Model file for the job. Use its own axes, mm. A direction names the side the tool comes from. Coordinates: 2 decimals unless noted, no trailing zeros. Write each loop counter-clockwise with the first axis right and the second up, starting at its lowest first coordinate (ties: lowest second). Pieces come first, ordered by that corner, then holes. Notation, with made-up numbers: M 74,80.5 L 82,80.5 A23 cw 82,102.5 Z; hole C 87,12 d4. An arc over 180 degrees is marked long. Put each result on its own line as item: value. Start each with the question number.
Q1. Cut at B-B (x = 305). Write the cut outline in (y, z), then the cut area to 3 significant figures.
Q2. Drop flat-ended pins along their axis: pin 1 (18 mm diameter, centred on x = 254, y = 25.4, fed in from -Z); pin 2 (1 mm diameter, centred on x = 383.5, y = 85, fed in from +Z); pin 3 (5.5 mm diameter, centred on x = 377.5, z = 27.5, fed in from +Y). Give the stop position or say it passes through.
Q3. Cut at A-A (z = -4). Write the cut outline in (x, y).
Q4. Which spindle directions (+Z, -Z, +X, -X, +Y, -Y) get a long thin tool onto all of the face, cutting with end or side? Do faces 1 (the flat face through (432, 26, 33.1)), 2 (the cylindrical face through (362.87, 87.91, 33.47)), 3 (the flat face through (341, 152.4, 0)), 4 (the flat face through (385, 50.8, 28)), 5 (the flat face through (344, 59, 38.1)). Say none if no direction does.
Q5. Pull direction Y, two halves, no side cores. Call faces 6 (the flat face through (341, 77, -38.1)), 7 (the flat face through (275.4, 75, 33)), 8 (the flat face through (341, 0, 0)), 9 (the flat face through (254, 26, 33.1)): pulls with the +Y half, pulls with the -Y half, needs draft (parallel to the pull), parting line crosses it, or undercut.
Q6. Drill centre lines: line 1 along Y through (x, z) = (254, 6.5); line 2 along X through (y, z) = (31, 13); line 3 along Y through (x, z) = (284.5, 35.5). Where is each one in solid material? Low to high.
Q7. Cut at D-D (z = 21.5). Write the cut outline in (x, y) (1 decimal).
Q8. Cut at C-C (y = 76.5). Write the cut outline in (x, z), then the cut area to 3 significant figures.
```python
from build123d import *

# Parameters (mm, degrees)
SALIENTE_EXTRUIR1_DEPTH = 19.05
SALIENTE_EXTRUIR2_DEPTH = 38.1
CROQUIS1_5_W            = 88.9
CROQUIS1_5_H            = 19.05
SALIENTE_EXTRUIR3_DEPTH = 28.702
CROQUIS2_W              = 42.1
CROQUIS2_H              = 101.6
CORTAR_EXTRUIR1_DEPTH   = 19.05
REDONDEO1_R             = 4.7625
CROQUIS4_W              = 84.9
CROQUIS4_H              = 38.1
SALIENTE_EXTRUIR4_DEPTH = 15.05
CROQUIS5_W              = 228.6
CROQUIS5_H              = 152.4
SALIENTE_EXTRUIR5_DEPTH = 38.1
REDONDEO2_R             = 2.54
CROQUIS6_R              = 10
CORTAR_EXTRUIR2_DEPTH   = 71.2
CROQUIS7_W              = 228.6
CROQUIS7_H              = 156.90491855
CORTAR_EXTRUIR3_DEPTH   = 488.918066892


with BuildPart() as part:
    # Croquis1 → Saliente-Extruir1 (new body)
    with BuildSketch(Plane.XY):
        Polygon((0, 0), (0, 152.4), (143.7, 152.4), (143.7, 137.35), (228.6, 137.35), (228.6, 0), align=None)
    extrude(amount=SALIENTE_EXTRUIR1_DEPTH)

    # Croquis1<4> → Saliente-Extruir2 (add)
    with BuildSketch(Plane.XY):
        Polygon((0, 152.4), (0, 0), (228.6, 0), (228.6, 137.35), (143.7, 137.35), (143.7, 152.4), (92.9, 152.4), (92.9, 86.55), (181.8, 86.55), (181.8, 63.5), (92.9, 63.5), (92.9, 50.8), (50.8, 50.8), (50.8, 152.4), align=None)
    extrude(amount=SALIENTE_EXTRUIR2_DEPTH)

    # Croquis1<5> → Saliente-Extruir3 (add)
    with BuildSketch(Plane.XY):
        with Locations((135.35, 75.025)):
            Rectangle(CROQUIS1_5_W, CROQUIS1_5_H)
        Polygon((92.9, 65.5), (92.9, 63.5), (181.8, 63.5), (181.8, 86.55), (92.9, 86.55), (92.9, 84.55), (179.8, 84.55), (179.8, 65.5), align=None)
    extrude(amount=SALIENTE_EXTRUIR3_DEPTH)

    # Croquis2 → Cortar-Extruir1 (cut)
    with BuildSketch(Plane.XY.offset(38.1)):
        with Locations((71.85, 101.6)):
            Rectangle(CROQUIS2_W, CROQUIS2_H)
    extrude(amount=-CORTAR_EXTRUIR1_DEPTH, mode=Mode.SUBTRACT)

    # Redondeo1
    redondeo1_edges = [part.edges().sort_by_distance(p)[0] for p in [
        (92.9, 86.55, 33.401),
        (181.8, 86.55, 33.401),
        (181.8, 63.5, 33.401),
        (92.9, 63.5, 33.401),
        (92.9, 50.8, 28.575),
        (50.8, 50.8, 28.575),
    ]]
    fillet(redondeo1_edges, radius=REDONDEO1_R)

    # Croquis4 → Saliente-Extruir4 (add)
    with BuildSketch(Plane(origin=(0, 137.35, 0), x_dir=(1, 0, 0), z_dir=(0, 1, 0))):
        with Locations((186.15, -19.05)):
            Rectangle(CROQUIS4_W, CROQUIS4_H)
    extrude(amount=SALIENTE_EXTRUIR4_DEPTH)

    # Croquis5 → Saliente-Extruir5 (add)
    with BuildSketch(Plane(origin=(0, 0, 0), x_dir=(-1, 0, 0), z_dir=(0, 0, -1))):
        with Locations((-114.3, 76.2)):
            Rectangle(CROQUIS5_W, CROQUIS5_H)
    extrude(amount=SALIENTE_EXTRUIR5_DEPTH)

    # Redondeo2
    redondeo2_edges = [part.edges().sort_by_distance(p)[0] for p in [
        (228.6, 0, 0),
        (0, 0, 0),
        (0, 152.4, 0),
        (228.6, 152.4, 0),
        (0, 76.2, -38.1),
        (114.3, 152.4, -38.1),
        (228.6, 76.2, -38.1),
        (114.3, 0, -38.1),
        (25.4, 152.4, 38.1),
        (0, 76.2, 38.1),
        (114.3, 0, 38.1),
        (228.6, 76.2, 38.1),
        (160.75, 152.4, 38.1),
    ]]
    fillet(redondeo2_edges, radius=REDONDEO2_R)

    # Croquis6 → Cortar-Extruir2 (cut)
    with BuildSketch(Plane(origin=(0, 0, -38.1), x_dir=(-1, 0, 0), z_dir=(0, 0, -1))):
        with Locations((-25.4, 127)):
            Circle(CROQUIS6_R)
        with Locations((-203.2, 127)):
            Circle(CROQUIS6_R)
        with Locations((-203.2, 25.4)):
            Circle(CROQUIS6_R)
        with Locations((-25.4, 25.4)):
            Circle(CROQUIS6_R)
        with Locations((-114.3, 25.4)):
            Circle(CROQUIS6_R)
    extrude(amount=-CORTAR_EXTRUIR2_DEPTH, mode=Mode.SUBTRACT)

    # Simetría1: part across plane


with BuildPart() as part_1:
    add(part.part)
    add(part.part.mirror(Plane(origin=(228.6, 0, 19.05), x_dir=(0, 0, 1), z_dir=(1, 0, 0))))

    # Croquis7 → Cortar-Extruir3 (cut, through all)
    with BuildSketch(Plane.XY.offset(38.1)):
        with Locations((114.3, 78.452459275)):
            Rectangle(CROQUIS7_W, CROQUIS7_H)
    extrude(amount=-CORTAR_EXTRUIR3_DEPTH, mode=Mode.SUBTRACT)


solid = part_1.part
```
Computed values:
1. outline: M 0,-35.56 A2.54 ccw 2.54,-38.1 L 149.86,-38.1 A2.54 ccw 152.4,-35.56 L 152.4,35.56 A2.54 ccw 149.86,38.1 L 86.55,38.1 L 86.55,28.7 L 63.5,28.7 L 63.5,38.1 L 2.54,38.1 A2.54 ccw 0,35.56 Z
1. area: 11,400 mm2
2. pin 1: z = 33.1
2. pin 2: z = 19.05
2. pin 3: y = 50.8
3. outline: M 228.6,2.54 A2.54 ccw 231.14,0 L 454.66,0 A2.54 ccw 457.2,2.54 L 457.2,149.86 A2.54 ccw 454.66,152.4 L 231.14,152.4 A2.54 ccw 228.6,149.86 Z; hole C 254,25.4 d20; hole C 254,127 d20; hole C 342.9,25.4 d20; hole C 431.8,25.4 d20; hole C 431.8,127 d20
4. face 1: -Z
4. face 2: +Z
4. face 3: +Z, -Z, +X, -X, +Y
4. face 4: +Z, +Y
4. face 5: +Z, +X, -X, +Y, -Y
5. face 6: needs draft
5. face 7: undercut
5. face 8: pulls with the -Y half
5. face 9: undercut
6. line 1: 0 to 15.4, 35.4 to 117, 137 to 152.4
6. line 2: 228.6 to 245.72, 262.28 to 334.62, 351.18 to 423.52, 440.08 to 457.2
6. line 3: 0 to 63.5, 86.55 to 152.4
7. outline: M 228.6,2.5 A2.5 ccw 231.1,0 L 454.7,0 A2.5 ccw 457.2,2.5 L 457.2,149.9 A2.5 ccw 454.7,152.4 L 406.4,152.4 L 406.4,55.6 A4.8 cw 401.6,50.8 L 369.1,50.8 A4.8 cw 364.3,55.6 L 364.3,152.4 L 231.1,152.4 A2.5 ccw 228.6,149.9 Z; hole C 254,25.4 d20; hole C 254,127 d20; hole C 342.9,25.4 d20; hole C 431.8,25.4 d20; hole C 431.8,127 d20
8. outline: M 228.6,-35.56 A2.54 ccw 231.14,-38.1 L 454.66,-38.1 A2.54 ccw 457.2,-35.56 L 457.2,35.56 A2.54 ccw 454.66,38.1 L 406.4,38.1 L 406.4,19.05 L 364.3,19.05 L 364.3,28.7 L 275.4,28.7 L 275.4,38.1 L 231.14,38.1 A2.54 ccw 228.6,35.56 Z
8. area: 15,800 mm2
